from build123d import *

# Parameters (mm, degrees)
SKETCH1_R           = 20
SKETCH1_R_2         = 5
BOSS_EXTRUDE1_DEPTH = 5
BOSS_EXTRUDE2_START = -1
SKETCH1_3_R         = 23
SKETCH1_3_R_2       = 20
SKETCH1_3_R_3       = 5
BOSS_EXTRUDE2_DEPTH = 1
BOSS_EXTRUDE3_START = 5
SKETCH1_4_R         = 23
SKETCH1_4_R_2       = 20
SKETCH1_4_R_3       = 5
BOSS_EXTRUDE3_DEPTH = 1


with BuildPart() as part:
    # Sketch1 → Boss-Extrude1 (new body)
    with BuildSketch(Plane(origin=(0, 0, 0), x_dir=(1, 0, 0), z_dir=(0, 1, 0))):
        with Locations(Location((0, 0, 0), (0, 0, 270))):
            Circle(SKETCH1_R)
        with Locations(Location((0, 0, 0), (0, 0, 270))):
            Circle(SKETCH1_R_2, mode=Mode.SUBTRACT)
    extrude(amount=BOSS_EXTRUDE1_DEPTH)

    # Sketch1<3> → Boss-Extrude2 (add)
    # profile 1 of 2: a face of its own
    with BuildSketch(Plane(origin=(0, 0, 0), x_dir=(1, 0, 0), z_dir=(0, 1, 0)).offset(BOSS_EXTRUDE2_START)):
        with Locations(Location((0, 0, 0), (0, 0, 270))):
            Circle(SKETCH1_3_R)
        with Locations(Location((0, 0, 0), (0, 0, 270))):
            Circle(SKETCH1_3_R_2, mode=Mode.SUBTRACT)
    # profile 2 of 2: a face of its own
    with BuildSketch(Plane(origin=(0, 0, 0), x_dir=(1, 0, 0), z_dir=(0, 1, 0)).offset(BOSS_EXTRUDE2_START)):
        with Locations(Location((0, 0, 0), (0, 0, 270))):
            Circle(SKETCH1_3_R_2)
        with Locations(Location((0, 0, 0), (0, 0, 270))):
            Circle(SKETCH1_3_R_3, mode=Mode.SUBTRACT)
    extrude(amount=BOSS_EXTRUDE2_DEPTH)

    # Sketch1<4> → Boss-Extrude3 (add)
    # profile 1 of 2: a face of its own
    with BuildSketch(Plane(origin=(0, 0, 0), x_dir=(1, 0, 0), z_dir=(0, 1, 0)).offset(BOSS_EXTRUDE3_START)):
        with Locations(Location((0, 0, 0), (0, 0, 270))):
            Circle(SKETCH1_4_R)
        with Locations(Location((0, 0, 0), (0, 0, 270))):
            Circle(SKETCH1_4_R_2, mode=Mode.SUBTRACT)
    # profile 2 of 2: a face of its own
    with BuildSketch(Plane(origin=(0, 0, 0), x_dir=(1, 0, 0), z_dir=(0, 1, 0)).offset(BOSS_EXTRUDE3_START)):
        with Locations(Location((0, 0, 0), (0, 0, 270))):
            Circle(SKETCH1_4_R_2)
        with Locations(Location((0, 0, 0), (0, 0, 270))):
            Circle(SKETCH1_4_R_3, mode=Mode.SUBTRACT)
    extrude(amount=BOSS_EXTRUDE3_DEPTH)


solid = part.part
Can you work these out from the model? Positions are in its coordinate system, mm. A direction names the side the tool comes from. Round coordinates to 2 decimals unless told otherwise and drop trailing zeros. Write each loop counter-clockwise with the first axis right and the second up, starting at its lowest first coordinate (ties: lowest second). Pieces come first, ordered by that corner, then holes. Notation, with made-up numbers: (-11, 26.5) -> (10, 26.5) arc R13 ccw to (10, 46.5) -> close; hole circle Ø4 at (56, 49.5). An arc over 180 degrees is marked (long way). Use one line per item in the form item = value. Start each with the question number.
Q1. Imagine slicing it at D-D (x = 14.5). Please give me the cut outline in (y, z), then the cut area to 3 significant figures.
Q2. Imagine slicing it at C-C (y = 1.75). Please give me the cut outline in (x, z).
Q3. We'd pull the mould along Y, two halves only. Please class faces 3 (the face through (19.394, 5.493, 12.365)), 4 (the face through (5.4, -1, -0.3)), 5 (the face through (19, 5, -7)): +Y half, -Y half, draft (parallel to the pull), parting line (faces both ways), or undercut.
Q4. Imagine slicing it at A-A (z = 0). Please give me the cut outline in (x, y), then the cut area to 3 significant figures.
Q5. I'm going to push flat-ended pins straight in: P1, Ø4, axis at x = -17.5, y = 0.5, coming from the +Z side; P2, Ø1.5, axis at y = 3.5, z = -5.5, coming from the +X side. Where does each tip first touch, or does it pass through?
Q6. If I drill on probe 1 along X at (y, z) = (1.75, 0); probe 2 along Y at (x, z) = (-12.5, -19); probe 3 along Z at (x, y) = (14, 1.25), over which ranges is the centre line in solid material (lowest first)? Write a range as [from, to].
Q7. Which directions (+Z, -Z, +X, -X, +Y, -Y) give clear straight access to the entire face, cutting with the end or side of a thin tool? Please do faces 1 (the face through (-4.88, 2.45, -1.08)), 2 (the face through (19, 0, -7)).
Q8. Imagine slicing it at B-B (x = 0). Please give me the cut outline in (y, z).
Worked out:
q1.outline = (-1, -17.85) -> (0, -17.85) -> (0, -13.77) -> (5, -13.77) -> (5, -17.85) -> (6, -17.85) -> (6, 17.85) -> (5, 17.85) -> (5, 13.77) -> (0, 13.77) -> (0, 17.85) -> (-1, 17.85) -> close
q1.area = 209 mm^2
q2.outline = circle Ø40 at (0, 0); hole circle Ø10 at (0, 0)
q3.face_3 = draft
q3.face_4 = -Y half
q3.face_5 = undercut
q4.outline = (-23, -1) -> (-5, -1) -> (-5, 6) -> (-23, 6) -> (-23, 5) -> (-20, 5) -> (-20, 0) -> (-23, 0) -> close; (5, -1) -> (23, -1) -> (23, 0) -> (20, 0) -> (20, 5) -> (23, 5) -> (23, 6) -> (5, 6) -> close
q4.area = 222 mm^2
q5.P1 = 16.93
q5.P2 = 19.43
q6.probe_1 = [-20, -5], [5, 20]
q6.probe_2 = [-1, 0], [5, 6]
q6.probe_3 = [-14.28, 14.28]
q7.face_1 = +Y, -Y
q7.face_2 = none
q8.outline = (-1, -23) -> (0, -23) -> (0, -20) -> (5, -20) -> (5, -23) -> (6, -23) -> (6, -5) -> (-1, -5) -> close; (-1, 5) -> (6, 5) -> (6, 23) -> (5, 23) -> (5, 20) -> (0, 20) -> (0, 23) -> (-1, 23) -> close
